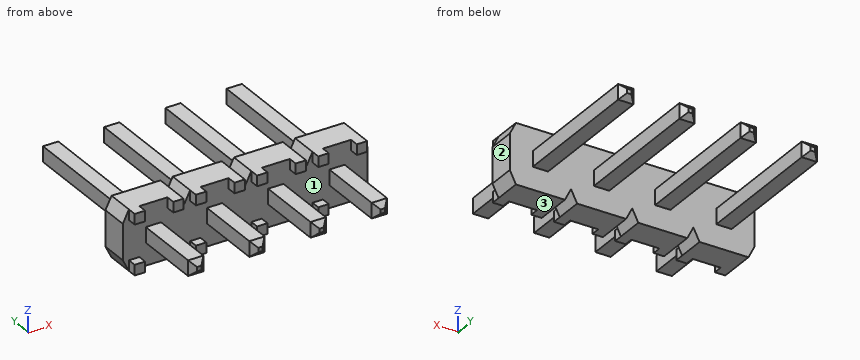
```python
from build123d import *

# Parameters (mm, degrees)
SKETCH1_W                        = 10.16
SKETCH1_H                        = 2.4892
BASE_EXTRUDE_DEPTH               = 0.5715
SNAP_GROOVES_DEPTH               = 2.143
SKETCH4_W                        = 0.4318
SKETCH4_H                        = 0.4318
STANDOFFS_DEPTH                  = 0.381
POSITION_PATTERN_COUNT           = 4
POSITION_PATTERN_PITCH           = 2.54
SKETCH5_W                        = 0.635
SKETCH5_H                        = 10
TERMINAL_TH_DEPTH                = 0.3175
T1_TIP1_SIZE                     = 0.2286
TERMINAL_PATTERN_COUNT           = 4
TERMINAL_PATTERN_PITCH           = 2.54
T1_TIP1_OF_TERMINAL_PATTERN_SIZE = 0.2286


with BuildPart() as part:
    # Sketch1 → Base-Extrude (new body, symmetric)
    with BuildSketch(Plane(origin=(0, 0, 0), x_dir=(1, 0, 0), z_dir=(0, 1, 0))):
        Rectangle(SKETCH1_W, SKETCH1_H)
    extrude(amount=BASE_EXTRUDE_DEPTH, both=True)

    # Sketch3 → Snap Grooves (cut, through all)
    with BuildSketch(Plane(origin=(0, 0.5715, 0), x_dir=(-1, 0, 0), z_dir=(0, 1, 0))):
        Polygon((2.286, 1.2446), (2.794, 1.2446), (2.54, 0.7366), align=None)
        Polygon((2.286, -1.2446), (2.794, -1.2446), (2.54, -0.7366), align=None)
        Polygon((5.08, -0.7366), (5.334, -1.2446), (4.826, -1.2446), align=None)
        Polygon((5.08, 0.7366), (5.334, 1.2446), (4.826, 1.2446), align=None)
    snap_grooves = extrude(amount=-SNAP_GROOVES_DEPTH, mode=Mode.SUBTRACT)

    # Sketch4 → Standoffs (add)
    with BuildSketch(Plane.XZ.offset(0.5715)):
        with Locations((-4.6101, 1.0287)):
            Rectangle(SKETCH4_W, SKETCH4_H)
        with Locations((-3.0099, 1.0287)):
            Rectangle(SKETCH4_W, SKETCH4_H)
        with Locations((-3.0099, -1.0287)):
            Rectangle(SKETCH4_W, SKETCH4_H)
        with Locations((-4.6101, -1.0287)):
            Rectangle(SKETCH4_W, SKETCH4_H)
    standoffs = extrude(amount=STANDOFFS_DEPTH)

    # Position Pattern: Snap Grooves, Standoffs ×4
    with Locations(*[(i * POSITION_PATTERN_PITCH, 0, 0) for i in range(1, POSITION_PATTERN_COUNT)]):
        add(snap_grooves, mode=Mode.SUBTRACT)
        add(standoffs)

    # Sketch5 → Terminal -TH (add, symmetric)
    with BuildSketch(Plane.ZY.offset(3.81)):
        with Locations((0, 1.4135)):
            Rectangle(SKETCH5_W, SKETCH5_H)
    terminal_th = extrude(amount=TERMINAL_TH_DEPTH, both=True)

    # T1 Tip1
    t1_tip1_edges = [part.edges().sort_by_distance(p)[0] for p in [
        (-3.81, -3.5865, 0.3175),
        (-4.1275, -3.5865, 0),
        (-3.81, 6.4135, -0.3175),
        (-3.4925, -3.5865, 0),
        (-3.81, -3.5865, -0.3175),
        (-3.4925, 6.4135, 0),
        (-3.81, 6.4135, 0.3175),
        (-4.1275, 6.4135, 0),
    ]]
    chamfer(t1_tip1_edges, length=T1_TIP1_SIZE)

    # Terminal Pattern: Terminal -TH ×4
    with Locations(*[(i * TERMINAL_PATTERN_PITCH, 0, 0) for i in range(1, TERMINAL_PATTERN_COUNT)]):
        add(terminal_th)

    # T1 Tip1 of Terminal Pattern
    t1_tip1_of_terminal_pattern_edges = [part.edges().sort_by_distance(p)[0] for p in [
        (-1.27, -3.5865, 0.3175),
        (-1.5875, -3.5865, 0),
        (-1.27, 6.4135, -0.3175),
        (-0.9525, -3.5865, 0),
        (-1.27, -3.5865, -0.3175),
        (-0.9525, 6.4135, 0),
        (-1.27, 6.4135, 0.3175),
        (-1.5875, 6.4135, 0),
        (1.27, -3.5865, 0.3175),
        (0.9525, -3.5865, 0),
        (1.27, 6.4135, -0.3175),
        (1.5875, -3.5865, 0),
        (1.27, -3.5865, -0.3175),
        (1.5875, 6.4135, 0),
        (1.27, 6.4135, 0.3175),
        (0.9525, 6.4135, 0),
        (3.81, -3.5865, 0.3175),
        (3.4925, -3.5865, 0),
        (3.81, 6.4135, -0.3175),
        (4.1275, -3.5865, 0),
        (3.81, -3.5865, -0.3175),
        (4.1275, 6.4135, 0),
        (3.81, 6.4135, 0.3175),
        (3.4925, 6.4135, 0),
    ]]
    chamfer(t1_tip1_of_terminal_pattern_edges, length=T1_TIP1_OF_TERMINAL_PATTERN_SIZE)


solid = part.part
```
Input: part model. Units: mm. Frame: model coordinates. Face numbers are marked on the shaded views. Round coordinates to 2 decimals unless told otherwise and drop trailing zeros. Loops run counter-clockwise (first coordinate to the right, second up) from the corner with the lowest first, then second, coordinate; pieces in that order, holes last. Notation, with made-up numbers: (8, 72.25) -> (17, 72.25) arc R11 cw to (17, 80.25) -> close; hole circle Ø1 at (1, 29). An arc over 180 degrees is marked (long way). Use one line per item in the form item = value. Start each with the question number.
Item 1: Mould query, pull axis Z, two halves, no side actions, for the marked faces 1, 2 and 3. Classes: pulls with the +Z half, pulls with the -Z half, needs draft (parallel to the pull), parting line crosses it, or undercut.
Item 2: Section query A-A on y = 0. Return the cut outline in (x, z), then the cut area to 3 significant figures.
Item 3: Contact query for flat-ended pins moving along their axis: pin 1 Ø0.7 at (x, y) = (-1, -2) entering from -Z; pin 2 Ø0.5 at (y, z) = (-2.5, 0) entering from -X; pin 3 Ø0.5 at (x, y) = (-4, 4) entering from +Z. Output: stop coordinate, or through.
Item 4: Section query C-C on y = 4.25. Return the cut outline in (x, z).
Item 5: Material intervals for L1, parallel to X at y = -0.75, z = 0.1; L2, parallel to X at y = 0.5, z = 1.15; L3, parallel to Y at x = -3.75, z = -0.85, sorted ascending. Write a range as from..to.
Item 6: Section query D-D on z = -0.6. Return the cut outline in (x, y).
Item 7: Section query B-B on x = 2. Return the cut outline in (y, z), then the cut area to 3 significant figures.
Ans:
q1.face_1 = undercut
q1.face_2 = needs draft
q1.face_3 = pulls with the -Z half
q2.outline = (-5.08, -0.74) -> (-4.83, -1.24) -> (-2.79, -1.24) -> (-2.54, -0.74) -> (-2.29, -1.24) -> (-0.25, -1.24) -> (0, -0.74) -> (0.25, -1.24) -> (2.29, -1.24) -> (2.54, -0.74) -> (2.79, -1.24) -> (4.83, -1.24) -> (5.08, -0.74) -> (5.08, 0.74) -> (4.83, 1.24) -> (2.79, 1.24) -> (2.54, 0.74) -> (2.29, 1.24) -> (0.25, 1.24) -> (0, 0.74) -> (-0.25, 1.24) -> (-2.29, 1.24) -> (-2.54, 0.74) -> (-2.79, 1.24) -> (-4.83, 1.24) -> (-5.08, 0.74) -> close
q2.area = 24.3 mm^2
q3.pin_1 = -0.32
q3.pin_2 = -4.13
q3.pin_3 = 0.32
q4.outline = (-4.13, -0.32) -> (-3.49, -0.32) -> (-3.49, 0.32) -> (-4.13, 0.32) -> close; (-1.59, -0.32) -> (-0.95, -0.32) -> (-0.95, 0.32) -> (-1.59, 0.32) -> close; (0.95, -0.32) -> (1.59, -0.32) -> (1.59, 0.32) -> (0.95, 0.32) -> close; (3.49, -0.32) -> (4.13, -0.32) -> (4.13, 0.32) -> (3.49, 0.32) -> close
q5.L1 = -4.13..-3.49, -1.59..-0.95, 0.95..1.59, 3.49..4.13
q5.L2 = -4.87..-2.75, -2.33..-0.21, 0.21..2.33, 2.75..4.87
q5.L3 = -0.57..0.57
q6.outline = (-5.08, -0.57) -> (5.08, -0.57) -> (5.08, 0.57) -> (-5.08, 0.57) -> close
q7.outline = (-0.95, -1.24) -> (0.57, -1.24) -> (0.57, 1.24) -> (-0.95, 1.24) -> (-0.95, 0.81) -> (-0.57, 0.81) -> (-0.57, -0.81) -> (-0.95, -0.81) -> close
q7.area = 3.17 mm^2
